Part print with two shaded views. Sizes in mm from the minimum x, y, z corner. Round coordinates to 2 decimals unless told otherwise and drop trailing zeros. Loops run counter-clockwise (first coordinate to the right, second up) from the corner with the lowest first, then second, coordinate; pieces in that order, holes last. Notation, with made-up numbers: M 87.5,62 L 92.5,62 A25 cw 92.5,90 Z; hole C 63.5,-10 d5. An arc over 180 degrees is marked long. Answer as CSV lines item,"result". Start each with the question number.
Item 1: Wall check: line 1 (X direction, y = 20, z = 69); line 2 (X direction, y = 21.5, z = 69.85) (3 decimals). Give the ranges that are in metal, low to high.
Item 2: Band-saw the part on A-A (z = 69.85). Give the cut face in (x, y) (3 decimals), and give its area (3 significant figures).
Item 3: Mould opens along X. For the marked faces 1, 2 and 3 say: pulls with the +X half, pulls with the -X half, needs draft (parallel to the pull), parting line crosses it, or undercut.
Item 4: Band-saw the part on C-C (y = 3). Give the cut face in (x, z) (3 decimals), and give its area (3 significant figures).
Item 5: Band-saw the part on B-B (x = 69.85). Give the cut face in (y, z) (3 decimals), and give its area (3 significant figures).
Item 6: Drop flat-ended pins along their axis: pin 1 Ø8 at (x, y) = (89.5, 20.5) entering from +Z; pin 2 Ø2 at (x, y) = (71, 6.5) entering from -Z; pin 3 Ø8 at (y, z) = (27, 118) entering from -X; pin 4 Ø17 at (x, z) = (69.85, 69.85) entering from -Y. Give the stop position or say it passes through.
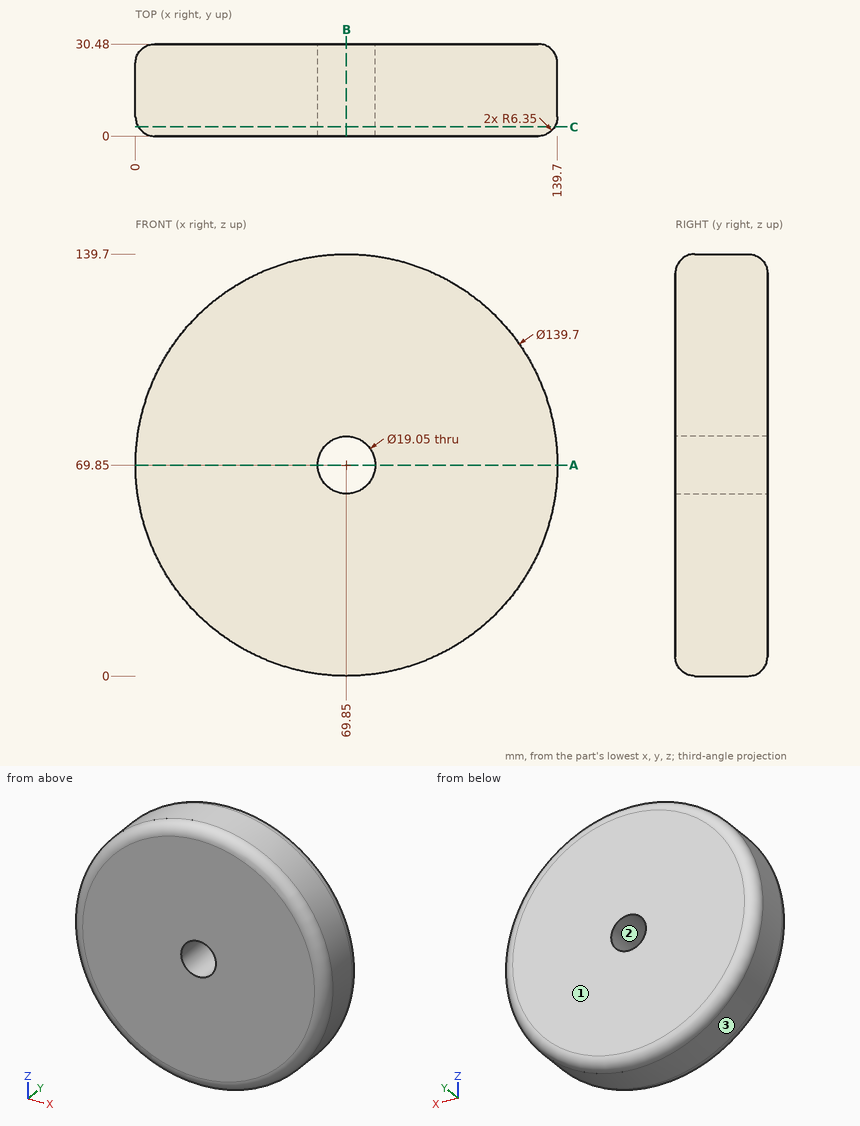
Answer block:
1,line 1,"x = 0.01 to 60.36, 79.34 to 139.69"
1,line 2,"x = 0 to 60.325, 79.375 to 139.7"
2,outline,"M 0,6.35 A6.35 ccw 6.35,0 L 60.325,0 L 60.325,30.48 L 6.35,30.48 A6.35 ccw 0,24.13 Z; M 79.375,0 L 133.35,0 A6.35 ccw 139.7,6.35 L 139.7,24.13 A6.35 ccw 133.35,30.48 L 79.375,30.48 Z"
2,area,"3,640 mm^2"
3,face 1,"needs draft"
3,face 2,"undercut"
3,face 3,"parting line crosses it"
4,outline,"C 69.85,69.85 d137.789; hole C 69.85,69.85 d19.05"
4,area,"14,600 mm^2"
5,outline,"M 0,6.35 A6.35 ccw 6.35,0 L 24.13,0 A6.35 ccw 30.48,6.35 L 30.48,60.325 L 0,60.325 Z; M 0,79.375 L 30.48,79.375 L 30.48,133.35 A6.35 ccw 24.13,139.7 L 6.35,139.7 A6.35 ccw 0,133.35 Z"
5,area,"3,640 mm^2"
6,pin 1,"stops at z = 137.92"
6,pin 2,"stops at z = 0"
6,pin 3,"stops at x = 16.15"
6,pin 4,"passes through"
